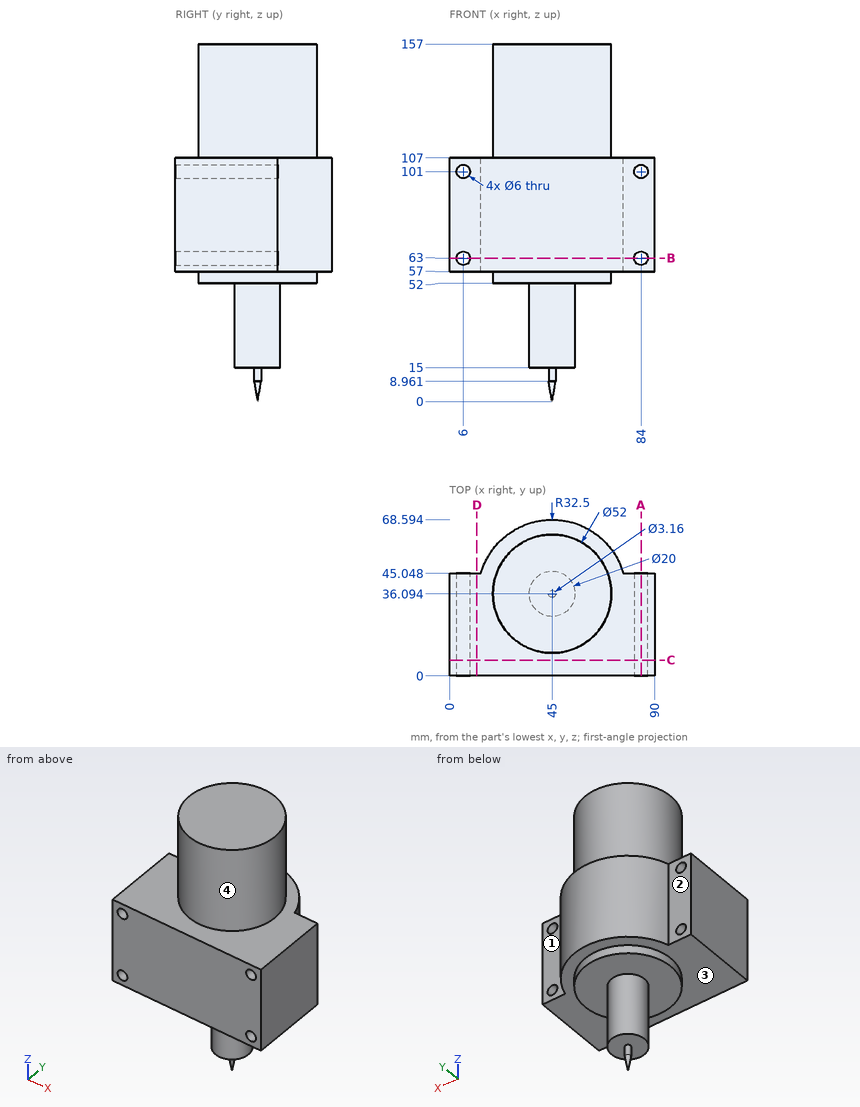
For this review, use the dimensioned drawing (mm, ordinates from the lowest corner) and the shaded views. A direction names the side the tool comes from. Give positions to 0.01 mm unless a question says otherwise; leave off trailing zeros. Loops run counter-clockwise (first coordinate to the right, second up) from the corner with the lowest first, then second, coordinate; pieces in that order, holes last.
Item 1: Take a section at A-A, the plane x = 84. State the section outline as (y, z) points, and give its area (3 significant figures).
Item 2: Insertion check: pin 1 (1 mm diameter, centred on x = 11.5, y = 33.5, fed in from -Z); pin 2 (3.5 mm diameter, centred on x = 6, z = 101, fed in from +Y); pin 3 (1 mm diameter, centred on x = 41.5, y = 36.5, fed in from -Z); pin 4 (8 mm diameter, centred on x = 40.5, z = 123.5, fed in from +Y). Each pin has a flat end and moves straight along its axis. Give the tip position at first contact, or say it passes through.
Item 3: Take a section at B-B, the plane z = 63. State the section outline as (x, y) points.
Item 4: For line 1 along Z through (x, y) = (6, 12); line 2 along Z through (x, y) = (83, 12); line 3 along Z through (x, y) = (45.5, 54), list the stretches that pass through material, from the lowest coordinate up.
Item 5: Take a section at D-D, the plane x = 12. State the section outline as (y, z) points, and give its area (3 significant figures).
Item 6: Take a section at C-C, the plane y = 7. State the section outline as (x, z) points.
Item 7: Tool access review of the marked faces 1, 2, 3 and 4: name each direction out of +Z, -Z, +X, -X, +Y, -Y from which nothing blocks a thin tool from reaching the whole face with its end or side.
Calculated:
1. outline: (0, 57) - (45.05, 57) - (45.05, 60) - (0, 60) - close; (0, 66) - (45.05, 66) - (45.05, 98) - (0, 98) - close; (0, 104) - (45.05, 104) - (45.05, 107) - (0, 107) - close
1. area: 1,710 mm2
2. pin 1: stops at z = 57
2. pin 2: passes through
2. pin 3: stops at z = 15
2. pin 4: stops at y = 62.09
3. outline: (0, 0) - (3, 0) - (3, 45.05) - (0, 45.05) - close; (9, 0) - (81, 0) - (81, 45.05) - (76.24, 45.05) arc R32.5 ccw to (13.76, 45.05) - (9, 45.05) - close; (87, 0) - (90, 0) - (90, 45.05) - (87, 45.05) - close
4. line 1: z = 57 to 60, 66 to 98, 104 to 107
4. line 2: z = 57 to 60.17, 65.83 to 98.17, 103.83 to 107
4. line 3: z = 52 to 157
5. outline: (0, 57) - (45.05, 57) - (45.05, 107) - (0, 107) - close
5. area: 2,250 mm2
6. outline: (0, 57) - (90, 57) - (90, 107) - (0, 107) - close; hole circle Ø6 at (6, 63); hole circle Ø6 at (6, 101); hole circle Ø6 at (84, 63); hole circle Ø6 at (84, 101)
7. face 1: +Z, -Z, +X, +Y
7. face 2: +Z, -Z, -X, +Y
7. face 3: -Z
7. face 4: +Z
